```python
from build123d import *

# Parameters (mm, degrees)
SKETCH1_W           = 38.1
SKETCH1_H           = 76.2
BOSS_EXTRUDE1_DEPTH = 6.35
SKETCH8_W           = 19.05
SKETCH8_H           = 76.2
BOSS_EXTRUDE5_DEPTH = 6.35
SKETCH5_R           = 6.604
BOSS_EXTRUDE2_DEPTH = 9.906
SKETCH6_R           = 3.302
CUT_EXTRUDE3_DEPTH  = 57.280347689
CUT_EXTRUDE4_START  = -1.27
SKETCH9_R           = 6.604
SKETCH9_R_2         = 5.207
CUT_EXTRUDE4_DEPTH  = 1.27
SKETCH11_W          = 38.1
SKETCH11_H          = 33.02
SKETCH11_R          = 2
BOSS_EXTRUDE6_DEPTH = 6.35


with BuildPart() as part:
    # Sketch1 → Boss-Extrude1 (new body)
    with BuildSketch(Plane.XY):
        Rectangle(SKETCH1_W, SKETCH1_H)
    extrude(amount=BOSS_EXTRUDE1_DEPTH)

    # Sketch8 → Boss-Extrude5 (add)
    with BuildSketch(Plane.XY.offset(6.35)):
        with Locations((-28.575, 0)):
            Rectangle(SKETCH8_W, SKETCH8_H)
        with Locations((28.575, 0)):
            Rectangle(SKETCH8_W, SKETCH8_H)
    extrude(amount=-BOSS_EXTRUDE5_DEPTH)

    # Sketch5 → Boss-Extrude2 (add)
    with BuildSketch(Plane.XY.offset(6.35)):
        with Locations(Location((22.86, 25.4, 0), (0, 0, 180))):
            Circle(SKETCH5_R)
        with Locations(Location((-22.86, 25.4, 0), (0, 0, 180))):
            Circle(SKETCH5_R)
    boss_extrude2 = extrude(amount=BOSS_EXTRUDE2_DEPTH)

    # Sketch6 → Cut-Extrude3 (cut, through all)
    with BuildSketch(Plane.XY.offset(16.256)):
        with Locations((22.86, 25.4)):
            Circle(SKETCH6_R)
        with Locations(Location((-22.86, 25.4, 0), (0, 0, 180))):
            Circle(SKETCH6_R)
    cut_extrude3 = extrude(amount=-CUT_EXTRUDE3_DEPTH, mode=Mode.SUBTRACT)

    # Sketch9 → Cut-Extrude4 (cut)
    # profile 1 of 2: a face of its own
    with BuildSketch(Plane.XY.offset(16.256).offset(CUT_EXTRUDE4_START)):
        with Locations(Location((-22.86, 25.4, 0), (0, 0, 180))):
            Circle(SKETCH9_R)
        with Locations((-22.86, 25.4)):
            Circle(SKETCH9_R_2, mode=Mode.SUBTRACT)
    # profile 2 of 2: a face of its own
    with BuildSketch(Plane.XY.offset(16.256).offset(CUT_EXTRUDE4_START)):
        with Locations(Location((22.86, 25.4, 0), (0, 0, 180))):
            Circle(SKETCH9_R)
        with Locations(Location((22.86, 25.4, 0), (0, 0, 180))):
            Circle(SKETCH9_R_2, mode=Mode.SUBTRACT)
    cut_extrude4 = extrude(amount=CUT_EXTRUDE4_DEPTH, mode=Mode.SUBTRACT)

    # Mirror1: Boss-Extrude2, Cut-Extrude3, Cut-Extrude4 across plane
    add(boss_extrude2.mirror(Plane.ZX))
    add(cut_extrude3.mirror(Plane.ZX), mode=Mode.SUBTRACT)
    add(cut_extrude4.mirror(Plane.ZX), mode=Mode.SUBTRACT)

    # Sketch11 → Boss-Extrude6 (add)
    with BuildSketch(Plane(origin=(0, 0, 0), x_dir=(-1, 0, 0), z_dir=(0, 0, -1))):
        with Locations((19.05, -54.61)):
            Rectangle(SKETCH11_W, SKETCH11_H)
        with Locations((6.35, -64.135)):
            Circle(SKETCH11_R, mode=Mode.SUBTRACT)
        with Locations((6.35, -45.085)):
            Circle(SKETCH11_R, mode=Mode.SUBTRACT)
    extrude(amount=-BOSS_EXTRUDE6_DEPTH)


solid = part.part
```
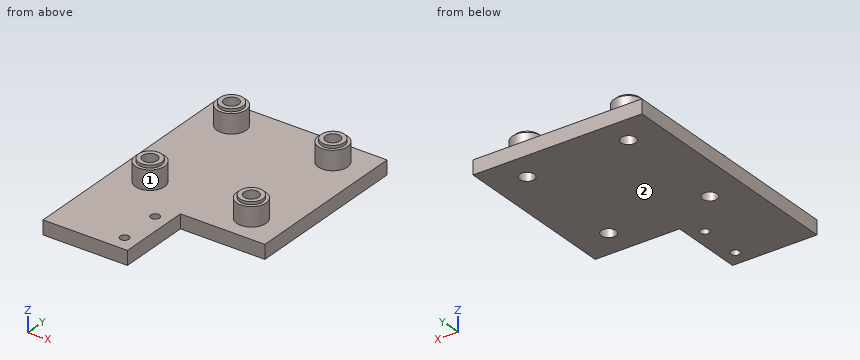
Source: CAD feature listing. Evaluate the final solid. Frame: model axes, mm. Face numbers are marked on the shaded views. Round coordinates to 2 decimals unless told otherwise and drop trailing zeros. Loops run counter-clockwise (first coordinate to the right, second up) from the corner with the lowest first, then second, coordinate; pieces in that order, holes last. Notation, with made-up numbers: M 1.5,56 L 8.5,56 A27 cw 8.5,86 Z; hole C 70,84 d10. An arc over 180 degrees is marked long. Use a Markdown table: item, result. Add a question column.
1. Line query: line 1 (Y direction, x = 22.86, z = 13.25); line 2 (Y direction, x = -6.35, z = 4.75) (3 decimals); line 3 (X direction, y = -45, z = 4.5). Output: solid intervals per line, ascending.
2. Contact query for flat-ended pins moving along their axis: P1, Ø5, axis at x = 16.5, z = 2, coming from the -Y side; P2, Ø12, axis at x = -14.5, y = 5, coming from the +Z side; P3, Ø8, axis at x = -20.5, z = 11.5, coming from the -Y side. Output: stop coordinate, or through.
3. Section query A-A on z = 9. Return the cut outline in (x, y), then the cut area to 3 significant figures.
4. Section query C-C on y = 25.4. Return the cut outline in (x, z).
5. Section query B-B on x = -22.86. Return the cut outline in (y, z), then the cut area to 3 significant figures.
6. Mould query, pull axis Y, two halves, no side actions, for the marked faces 1 and 2. Classes: pulls with the +Y half, pulls with the -Y half, needs draft (parallel to the pull), parting line crosses it, or undercut.
7. Section query D-D on z = 2.25. Return the cut outline in (x, y) (3 decimals).
Reported:
| question | item | result |
|---|---|---|
| 1 | line 1 | y = -32 to -28.7, -22.1 to -18.8, 18.8 to 22.1, 28.7 to 32 |
| 1 | line 2 | y = -71.12 to -66.135, -62.135 to -47.085, -43.085 to 38.1 |
| 1 | line 3 | x = -38.1 to -8.35, -4.35 to 0 |
| 2 | P1 | stops at y = -38.1 |
| 2 | P2 | stops at z = 6.35 |
| 2 | P3 | stops at y = -32 |
| 3 | outline | C -22.86,-25.4 d13.21; C -22.86,25.4 d13.21; C 22.86,-25.4 d13.21; C 22.86,25.4 d13.21; hole C -22.86,-25.4 d6.6; hole C -22.86,25.4 d6.6; hole C 22.86,-25.4 d6.6; hole C 22.86,25.4 d6.6 |
| 3 | area | 411 mm² |
| 4 | outline | M -38.1,0 L -26.16,0 L -26.16,16.26 L -28.07,16.26 L -28.07,14.99 L -29.46,14.99 L -29.46,6.35 L -38.1,6.35 Z; M -19.56,0 L 19.56,0 L 19.56,16.26 L 17.65,16.26 L 17.65,14.99 L 16.26,14.99 L 16.26,6.35 L -16.26,6.35 L -16.26,14.99 L -17.65,14.99 L -17.65,16.26 L -19.56,16.26 Z; M 26.16,0 L 38.1,0 L 38.1,6.35 L 29.46,6.35 L 29.46,14.99 L 28.07,14.99 L 28.07,16.26 L 26.16,16.26 Z |
| 5 | outline | M -71.12,0 L -28.7,0 L -28.7,16.26 L -30.61,16.26 L -30.61,14.99 L -32,14.99 L -32,6.35 L -71.12,6.35 Z; M -22.1,0 L 22.1,0 L 22.1,16.26 L 20.19,16.26 L 20.19,14.99 L 18.8,14.99 L 18.8,6.35 L -18.8,6.35 L -18.8,14.99 L -20.19,14.99 L -20.19,16.26 L -22.1,16.26 Z; M 28.7,0 L 38.1,0 L 38.1,6.35 L 32,6.35 L 32,14.99 L 30.61,14.99 L 30.61,16.26 L 28.7,16.26 Z |
| 5 | area | 733 mm² |
| 6 | face 1 | undercut |
| 6 | face 2 | needs draft |
| 7 | outline | M -38.1,-71.12 L 0,-71.12 L 0,-38.1 L 38.1,-38.1 L 38.1,38.1 L -38.1,38.1 Z; hole C -22.86,-25.4 d6.604; hole C -22.86,25.4 d6.604; hole C -6.35,-64.135 d4; hole C -6.35,-45.085 d4; hole C 22.86,-25.4 d6.604; hole C 22.86,25.4 d6.604 |
